from build123d import *

# Parameters (mm, degrees)
SKETCH_1_R          = 1.6
EXTRUDE_1_DEPTH     = 3
SKETCH_2_W          = 10
SKETCH_2_H          = 10
EXTRUDE_3_DEPTH     = 140
EXTRUDE_4_DEPTH     = 10
EXTRUDE_5_DEPTH     = 10
EXTRUDE_6_DEPTH     = 10
SKETCH_9_W          = 10
SKETCH_9_H          = 10
EXTRUDE_7_DEPTH     = 60
SKETCH_10_W         = 10
SKETCH_10_H         = 10
EXTRUDE_8_DEPTH     = 60
SKETCH_11_R         = 1.6
CUT_EXTRUDE_3_DEPTH = 20
SKETCH_12_R         = 1.6
CUT_EXTRUDE_4_DEPTH = 20


with BuildPart() as part:
    # 草图1 → 凸台-拉伸1 (new body)
    with BuildSketch(Plane.XY):
        with BuildLine():
            Line((33.5, 21.5), (-33.5, 21.5))
            ThreePointArc((-33.5, 21.5), (-35.621320344, 20.621320344), (-36.5, 18.5))
            Line((-36.5, 18.5), (-36.5, -18.5))
            ThreePointArc((-36.5, -18.5), (-35.621320344, -20.621320344), (-33.5, -21.5))
            Line((-33.5, -21.5), (33.5, -21.5))
            ThreePointArc((33.5, -21.5), (35.621320344, -20.621320344), (36.5, -18.5))
            Line((36.5, -18.5), (36.5, 18.5))
            ThreePointArc((36.5, 18.5), (35.621320344, 20.621320344), (33.5, 21.5))
        make_face()
        with Locations((33.5, 18.5)):
            Circle(SKETCH_1_R, mode=Mode.SUBTRACT)
        with Locations((-33.5, 18.5)):
            Circle(SKETCH_1_R, mode=Mode.SUBTRACT)
        with Locations(Location((33.5, -18.5, 0), (0, 0, 180))):
            Circle(SKETCH_1_R, mode=Mode.SUBTRACT)
        with Locations(Location((-33.5, -18.5, 0), (0, 0, 180))):
            Circle(SKETCH_1_R, mode=Mode.SUBTRACT)
        with BuildLine():
            Line((1.450268103, -4.227949809), (11.673904999, -9.873838841))
            ThreePointArc((11.673904999, -9.873838841), (13.1286742, -13.248837941), (10.223636896, -15.5))
            Line((10.223636896, -15.5), (-10.223636896, -15.5))
            ThreePointArc((-10.223636896, -15.5), (-13.1286742, -13.248837941), (-11.673904999, -9.873838841))
            Line((-11.673904999, -9.873838841), (-1.450268103, -4.227949809))
            ThreePointArc((-1.450268103, -4.227949809), (0, -3.854110968), (1.450268103, -4.227949809))
        make_face(mode=Mode.SUBTRACT)
        with BuildLine():
            Line((11.673904999, 9.873838841), (1.450268103, 4.227949809))
            ThreePointArc((1.450268103, 4.227949809), (0, 3.854110968), (-1.450268103, 4.227949809))
            Line((-1.450268103, 4.227949809), (-11.673904999, 9.873838841))
            ThreePointArc((-11.673904999, 9.873838841), (-13.1286742, 13.248837941), (-10.223636896, 15.5))
            Line((-10.223636896, 15.5), (10.223636896, 15.5))
            ThreePointArc((10.223636896, 15.5), (13.1286742, 13.248837941), (11.673904999, 9.873838841))
        make_face(mode=Mode.SUBTRACT)
    extrude(amount=EXTRUDE_1_DEPTH)

    # 草图2 → 凸台-拉伸3 (add)
    with BuildSketch(Plane.XY.offset(3)):
        with Locations((-22.5, 0)):
            Rectangle(SKETCH_2_W, SKETCH_2_H)
        with Locations((22.5, 0)):
            Rectangle(SKETCH_2_W, SKETCH_2_H)
    extrude(amount=EXTRUDE_3_DEPTH)

    # 草图5 → 凸台-拉伸4 (add)
    with BuildSketch(Plane.ZY.offset(27.5)):
        Polygon((3, 18.5), (3, 5), (143, 5), align=None)
    extrude(amount=-EXTRUDE_4_DEPTH)

    # 草图6 → 凸台-拉伸5 (add)
    with BuildSketch(Plane.ZY.offset(27.5)):
        Polygon((3, -5), (3, -18.5), (143, -5), align=None)
    extrude(amount=-EXTRUDE_5_DEPTH)

    # 草图7 → 凸台-拉伸6 (add)
    with BuildSketch(Plane(origin=(27.5, 0, 0), x_dir=(0, 0, -1), z_dir=(1, 0, 0))):
        Polygon((-143, 5), (-3, 5), (-3, 18.5), align=None)
        Polygon((-143, -5), (-3, -18.5), (-3, -5), align=None)
    extrude(amount=-EXTRUDE_6_DEPTH)

    # 草图9 → 凸台-拉伸7 (add)
    with BuildSketch(Plane.XY.offset(143)):
        with Locations((-22.5, 0)):
            Rectangle(SKETCH_9_W, SKETCH_9_H)
    extrude(amount=EXTRUDE_7_DEPTH)

    # 草图10 → 凸台-拉伸8 (add)
    with BuildSketch(Plane.XY.offset(143)):
        with Locations((22.5, 0)):
            Rectangle(SKETCH_10_W, SKETCH_10_H)
    extrude(amount=EXTRUDE_8_DEPTH)

    # 草图11 → 切除-拉伸3 (cut)
    with BuildSketch(Plane.XY.offset(203)):
        with Locations((-22.5, 0)):
            Circle(SKETCH_11_R)
    extrude(amount=-CUT_EXTRUDE_3_DEPTH, mode=Mode.SUBTRACT)

    # 草图12 → 切除-拉伸4 (cut)
    with BuildSketch(Plane.XY.offset(203)):
        with Locations((22.5, 0)):
            Circle(SKETCH_12_R)
    extrude(amount=-CUT_EXTRUDE_4_DEPTH, mode=Mode.SUBTRACT)


solid = part.part
Can you work these out from the model? Positions are in its coordinate system, mm. A direction names the side the tool comes from. Round coordinates to 2 decimals unless told otherwise and drop trailing zeros. Loops run counter-clockwise (first coordinate to the right, second up) from the corner with the lowest first, then second, coordinate; pieces in that order, holes last. Notation, with made-up numbers: (15.25, 59.5) - (57.25, 59.5) arc R7 ccw to (57.25, 68.5) - close; hole circle Ø10 at (53.25, 52). An arc over 180 degrees is marked (long way). Use CSV: the item, a comma, the result in double quotes. Start each with the question number.
1) If we section it at C-C on z = 60: Write out the boundary of the cut face in (x, y), plus the area to 3 significant figures.
2) If we section it at A-A on z = 176: Write out the boundary of the cut face in (x, y).
3) If we section it at B-B on x = 5.5: Write out the boundary of the cut face in (y, z), plus the area to 3 significant figures.
4) For faces 1 (the flat face through (22, -5, 173)), 2 (the flat face through (-1, 0, 0)), 3 (the flat face through (-23, 5, 173)), 4 (the flat face through (6.49, -7.01, 1.48)), 5 (the flat face through (-17.5, 0, 79)), which set-ups out of +Z, -Z, +X, -X, +Y, -Y let a thin tool reach every point of the face, with its end or its side?
5) Please list where these lines run through material, in increasing order: probe 1 along Y at (x, z) = (33.5, 1.8); probe 2 along X at (y, z) = (-18.5, 1.4); probe 3 along X at (y, z) = (-3, 15.5). Write a range as [from, to].
6) For pin 1 Ø1 at (x, y) = (-22.5, 0) entering from +Z; pin 2 Ø6 at (x, z) = (12.5, 122) entering from -Y; pin 3 Ø1 at (y, z) = (5, 169) entering from -X; pin 4 Ø3 at (x, z) = (20.5, 174) entering from +Y, each with a flat end and sliding along its axis, tell me the tip position at first contact or that it passes through.
7) We'd pull the mould along Y, two halves only. Please class faces 6 (the flat face through (-27.5, 0, 79)), 7 (the flat face through (6.63, 7.09, 1.48)), 8 (the flat face through (-22.57, -11.844, 72.02)): released by +Y, released by -Y, zero draft, split by the parting line, or undercut.
Geometry results:
1,outline,"(-27.5, -13) - (-17.5, -13) - (-17.5, 13) - (-27.5, 13) - close; (17.5, -13) - (27.5, -13) - (27.5, 13) - (17.5, 13) - close"
1,area,"520 mm2"
2,outline,"(-27.5, -5) - (-17.5, -5) - (-17.5, 5) - (-27.5, 5) - close; (17.5, -5) - (27.5, -5) - (27.5, 5) - (17.5, 5) - close"
3,outline,"(-21.5, 0) - (-15.5, 0) - (-15.5, 3) - (-21.5, 3) - close; (-6.46, 0) - (6.46, 0) - (6.46, 3) - (-6.46, 3) - close; (15.5, 0) - (21.5, 0) - (21.5, 3) - (15.5, 3) - close"
3,area,"74.8 mm2"
4,face 1,"+Z, +X, -X, -Y"
4,face 2,"-Z, +X, -X, +Y, -Y"
4,face 3,"+Z, +X, -X, +Y"
4,face 4,"+Z, -Z"
4,face 5,"+Z, +Y, -Y"
5,probe 1,"y = [-21.5, -20.1], [-16.9, 16.9], [20.1, 21.5]"
5,probe 2,"x = [-36.5, -35.1], [-31.9, 31.9], [35.1, 36.5]"
5,probe 3,"x = [-27.5, -17.5], [17.5, 27.5]"
6,pin 1,"stops at z = 183"
6,pin 2,"passes through"
6,pin 3,"stops at x = -27.5"
6,pin 4,"stops at y = 5"
7,face 6,"zero draft"
7,face 7,"undercut"
7,face 8,"released by -Y"
